from build123d import *

# Parameters (mm, degrees)
SKETCH1_R           = 1.524000008
SKETCH1_R_2         = 1.523999992
BOSS_EXTRUDE1_DEPTH = 1.575


with BuildPart() as part:
    # Sketch1 → Boss-Extrude1 (new body)
    with BuildSketch(Plane(origin=(0, 0, 0), x_dir=(1, 0, 0), z_dir=(0, 1, 0))):
        with BuildLine():
            Line((38.851293305, -40.014412246), (36.727293315, -40.014412246))
            Line((36.727293315, -40.014412246), (36.727293315, -40.012412246))
            Line((36.727293315, -40.012412246), (30.377293307, -40.012412246))
            Line((30.377293307, -40.012412246), (-29.674706693, -40.012412246))
            Line((-29.674706693, -40.012412246), (-36.024706701, -40.012412246))
            Line((-36.024706701, -40.012412246), (-36.024706701, -40.014412246))
            Line((-36.024706701, -40.014412246), (-40.148706691, -40.014412246))
            Line((-40.148706691, -40.014412246), (-40.148706691, -30.885946892))
            ThreePointArc((-40.148706691, -30.885946892), (-39.776732303, -29.98792128), (-38.878706691, -29.615946892))
            Line((-38.878706691, -29.615946892), (-34.543706691, -29.615946892))
            ThreePointArc((-34.543706691, -29.615946892), (-33.645681079, -29.243972504), (-33.273706691, -28.345946892))
            Line((-33.273706691, -28.345946892), (-33.273706691, -10.370428445))
            Line((-33.273706691, -10.370428445), (-12.148706691, -10.370428445))
            Line((-12.148706691, -10.370428445), (-12.148706691, -17.871301308))
            Line((-12.148706691, -17.871301308), (-12.148706691, -34.615947016))
            Line((-12.148706691, -34.615947016), (12.851293309, -34.615947016))
            Line((12.851293309, -34.615947016), (12.851293309, -17.871301308))
            Line((12.851293309, -17.871301308), (12.851293309, -10.370428445))
            Line((12.851293309, -10.370428445), (33.976293305, -10.370428445))
            Line((33.976293305, -10.370428445), (33.976293305, -28.345946892))
            ThreePointArc((33.976293305, -28.345946892), (34.348267693, -29.243972504), (35.246293305, -29.615946892))
            Line((35.246293305, -29.615946892), (38.851293305, -29.615946892))
            ThreePointArc((38.851293305, -29.615946892), (40.265506868, -30.20173333), (40.851293305, -31.615946892))
            Line((40.851293305, -31.615946892), (40.851293305, -38.014412246))
            ThreePointArc((40.851293305, -38.014412246), (40.265506868, -39.428625809), (38.851293305, -40.014412246))
        make_face()
        with Locations(Location((-36.024706701, -35.965946892, 0), (0, 0, 270))):
            Circle(SKETCH1_R, mode=Mode.SUBTRACT)
        with Locations(Location((36.727293315, -35.947946892, 0), (0, 0, 270))):
            Circle(SKETCH1_R_2, mode=Mode.SUBTRACT)
    extrude(amount=BOSS_EXTRUDE1_DEPTH)


solid = part.part
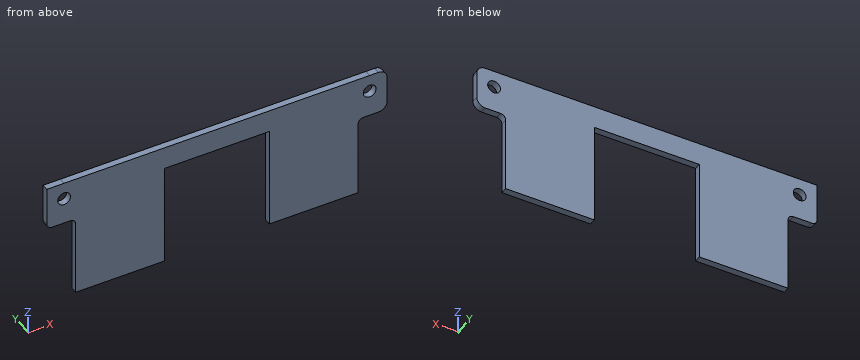
Input: part model. Units: mm. Frame: model coordinates. Coordinates: 2 decimals unless noted, no trailing zeros. Order: outer loops, then holes, each group sorted by start corner. A loop starts at its lowest first (then second) coordinate and runs counter-clockwise, first axis right, second up.
1. Cut plane A-A, the plane z = 22. Return loops of the section in (x, y) (3 decimals), plus the area to 3 significant figures.
Checked values:
outline: (-33.274, 0) - (-12.149, 0) - (-12.149, 1.575) - (-33.274, 1.575) - close; (12.851, 0) - (33.976, 0) - (33.976, 1.575) - (12.851, 1.575) - close
area: 66.5 mm2
2. Contact query for flat-ended pins moving along their axis: P1, Ø0.5, axis at y = 0.5, z = 18.5, coming from the -X side; P2, Ø0.8, axis at y = 1, z = 19.5, coming from the +X side; P3, Ø0.8, axis at x = 2.5, y = 0.5, coming from the -Z side; P4, Ø4, axis at x = -36.02, z = 35.97, coming from the -Y side. Output: stop coordinate, or through.
Checked values:
P1: stops at x = -33.27
P2: stops at x = 33.98
P3: stops at z = 34.62
P4: stops at y = 0
3. Cut plane C-C, the plane x = 11. Return loops of the section in (y, z) (3 decimals), plus the area to 3 significant figures.
Checked values:
outline: (0, 34.616) - (1.575, 34.616) - (1.575, 40.012) - (0, 40.012) - close
area: 8.50 mm2
4. Cut plane B-B, the plane y = 0.7. Count the separate pieces of the cut face and the enclosed holes in it, plus the area to 3 significant figures.
Checked values:
separate pieces: 1
enclosed holes: 2
area: 1,510 mm2
5. Ray query, line 1 along X through (y, z) = (0.75, 26); line 2 along X through (y, z) = (1.05, 36.5); line 3 along X through (y, z) = (1.2, 36.25). Return the intervals inside material, ascending.
Checked values:
line 1: x = -33.27 to -12.15, 12.85 to 33.98
line 2: x = -40.15 to -37.45, -34.6 to 35.31, 38.15 to 40.85
line 3: x = -40.15 to -37.52, -34.53 to 35.23, 38.22 to 40.85
